from build123d import *

# Parameters (mm, degrees)
SKETCH_1_W          = 106
SKETCH_1_H          = 103
SKETCH_1_W_2        = 102
SKETCH_1_H_2        = 99
EXTRUDE_1_DEPTH     = 25
SKETCH_2_W          = 106
SKETCH_2_H          = 103
EXTRUDE_2_DEPTH     = 1.4
SKETCH_3_R          = 3
SKETCH_3_R_2        = 1.35
EXTRUDE_3_DEPTH     = 5
SKETCH_4_W          = 12.8
SKETCH_4_H          = 11.5
CUT_EXTRUDE_1_DEPTH = 101
FILLET_1_R          = 2
CHAMFER_1_SIZE      = 1
SKETCH_5_R          = 4
SKETCH_5_R_2        = 5
CUT_EXTRUDE_2_DEPTH = 2
SKETCH_6_W          = 3
SKETCH_6_H          = 10
CUT_EXTRUDE_3_DEPTH = 2
SKETCH_8_R          = 1.5
CUT_EXTRUDE_4_DEPTH = 121.470950855
SKETCH_9_R          = 1.5
CUT_EXTRUDE_5_DEPTH = 2
SKETCH_10_W         = 10.5
SKETCH_10_H         = 3
CUT_EXTRUDE_6_DEPTH = 2


with BuildPart() as part:
    # Эскиз1 → Бобышка-Вытянуть1 (new body)
    with BuildSketch(Plane.XY):
        Rectangle(SKETCH_1_W, SKETCH_1_H)
        Rectangle(SKETCH_1_W_2, SKETCH_1_H_2, mode=Mode.SUBTRACT)
    extrude(amount=EXTRUDE_1_DEPTH)

    # Эскиз2 → Бобышка-Вытянуть2 (add)
    with BuildSketch(Plane(origin=(0, 0, 0), x_dir=(-1, 0, 0), z_dir=(0, 0, -1))):
        Rectangle(SKETCH_2_W, SKETCH_2_H)
    extrude(amount=EXTRUDE_2_DEPTH)

    # Эскиз3 → Бобышка-Вытянуть3 (add)
    # profile 1 of 4: a face of its own
    with BuildSketch(Plane.XY):
        with Locations(Location((-45, 39.5, 0), (0, 0, 180))):
            Circle(SKETCH_3_R)
        with Locations((-45, 39.5)):
            Circle(SKETCH_3_R_2, mode=Mode.SUBTRACT)
    # profile 2 of 4: a face of its own
    with BuildSketch(Plane.XY):
        with Locations(Location((45, 39.5, 0), (0, 0, 180))):
            Circle(SKETCH_3_R)
        with Locations((45, 39.5)):
            Circle(SKETCH_3_R_2, mode=Mode.SUBTRACT)
    # profile 3 of 4: a face of its own
    with BuildSketch(Plane.XY):
        with Locations(Location((-45, -43.5, 0), (0, 0, 180))):
            Circle(SKETCH_3_R)
        with Locations((-45, -43.5)):
            Circle(SKETCH_3_R_2, mode=Mode.SUBTRACT)
    # profile 4 of 4: a face of its own
    with BuildSketch(Plane.XY):
        with Locations(Location((45, -43.5, 0), (0, 0, 180))):
            Circle(SKETCH_3_R)
        with Locations((45, -43.5)):
            Circle(SKETCH_3_R_2, mode=Mode.SUBTRACT)
    extrude(amount=EXTRUDE_3_DEPTH)

    # Эскиз4 → Вырез-Вытянуть1 (cut)
    with BuildSketch(Plane.XZ.offset(51.5)):
        with Locations((10.1, 12.35)):
            Rectangle(SKETCH_4_W, SKETCH_4_H)
    extrude(amount=-CUT_EXTRUDE_1_DEPTH, mode=Mode.SUBTRACT)

    # Скругление1
    fillet_1_edges = [part.edges().sort_by_distance(p)[0] for p in [
        (51, -49.5, 12.5),
        (51, 49.5, 12.5),
        (-51, 49.5, 12.5),
        (-51, -49.5, 12.5),
        (53, -51.5, 11.8),
        (-53, -51.5, 11.8),
        (-53, 51.5, 11.8),
        (53, 51.5, 11.8),
    ]]
    fillet(fillet_1_edges, radius=FILLET_1_R)

    # Фаска1
    chamfer_1_edges = [part.edges().sort_by_distance(p)[0] for p in [
        (-51, 0, 0),
        (0, -49.5, 0),
        (51, 0, 0),
        (0, 49.5, 0),
        (50.414213562, -48.914213562, 0),
        (50.414213562, 48.914213562, 0),
        (-50.414213562, 48.914213562, 0),
        (-50.414213562, -48.914213562, 0),
        (-42, 39.5, 0),
        (48, 39.5, 0),
        (-42, -43.5, 0),
        (48, -43.5, 0),
    ]]
    chamfer(chamfer_1_edges, length=CHAMFER_1_SIZE)

    # Эскиз5 → Вырез-Вытянуть2 (cut)
    with BuildSketch(Plane.XZ.offset(51.5)):
        with Locations(Location((32.5, 14.6, 0), (0, 0, 270))):
            Circle(SKETCH_5_R)
        with Locations(Location((-8.3, 14.6, 0), (0, 0, 270))):
            Circle(SKETCH_5_R_2)
    extrude(amount=-CUT_EXTRUDE_2_DEPTH, mode=Mode.SUBTRACT)

    # Эскиз6 → Вырез-Вытянуть3 (cut)
    with BuildSketch(Plane(origin=(53, 0, 0), x_dir=(0, 0, -1), z_dir=(1, 0, 0))):
        with Locations((-23.5, -18.5)):
            Rectangle(SKETCH_6_W, SKETCH_6_H)
        with Locations((-23.5, 7.5)):
            Rectangle(SKETCH_6_W, SKETCH_6_H)
    extrude(amount=-CUT_EXTRUDE_3_DEPTH, mode=Mode.SUBTRACT)

    # Эскиз8 → Вырез-Вытянуть4 (cut, through all)
    with BuildSketch(Plane(origin=(53, 0, 0), x_dir=(0, 0, -1), z_dir=(1, 0, 0))):
        with Locations((-21, 43.5)):
            Circle(SKETCH_8_R)
        with Locations((-21, -43.5)):
            Circle(SKETCH_8_R)
    extrude(amount=-CUT_EXTRUDE_4_DEPTH, mode=Mode.SUBTRACT)

    # Эскиз9 → Вырез-Вытянуть5 (cut)
    with BuildSketch(Plane(origin=(53, 0, 0), x_dir=(0, 0, -1), z_dir=(1, 0, 0))):
        with Locations((-21, -5.5)):
            Circle(SKETCH_9_R)
    extrude(amount=-CUT_EXTRUDE_5_DEPTH, mode=Mode.SUBTRACT)

    # Эскиз10 → Вырез-Вытянуть6 (cut)
    with BuildSketch(Plane(origin=(0, 51.5, 0), x_dir=(1, 0, 0), z_dir=(0, 1, 0))):
        with Locations((9.75, -23.5)):
            Rectangle(SKETCH_10_W, SKETCH_10_H)
    extrude(amount=-CUT_EXTRUDE_6_DEPTH, mode=Mode.SUBTRACT)


solid = part.part
Here's how the part is built. I have some questions about the finished solid (model axes, mm). A direction names the side the tool comes from. Coordinates: 2 decimals unless noted, no trailing zeros. Write each loop counter-clockwise with the first axis right and the second up, starting at its lowest first coordinate (ties: lowest second). Pieces come first, ordered by that corner, then holes. Notation, with made-up numbers: (24, 89.5) - (31, 89.5) arc R26 cw to (31, 120.5) - close; hole circle Ø9 at (43, 49). An arc over 180 degrees is marked (long way). Use one line per item in the form item = value.
1) Suppose I cut it at B-B, the plane y = -5.5. Write out the boundary of the cut face in (x, z), plus the area to 3 significant figures.
Solved:
outline = (-53, -1.4) - (53, -1.4) - (53, 19.5) - (51, 19.5) - (51, 1) - (50, 0) - (-50, 0) - (-51, 1) - (-51, 25) - (-53, 25) - close; (51, 22.5) - (53, 22.5) - (53, 25) - (51, 25) - close
area = 243 mm2
2) Suppose I cut it at A-A, the plane z = 14.6. Write out the boundary of the cut face in (x, y).
Solved:
outline = (-53, -49.5) arc R2 ccw to (-51, -51.5) - (-13.3, -51.5) - (-13.3, -49.5) - (-49, -49.5) arc R2 cw to (-51, -47.5) - (-51, 47.5) arc R2 cw to (-49, 49.5) - (49, 49.5) arc R2 cw to (51, 47.5) - (51, -47.5) arc R2 cw to (49, -49.5) - (36.5, -49.5) - (36.5, -51.5) - (51, -51.5) arc R2 ccw to (53, -49.5) - (53, 49.5) arc R2 ccw to (51, 51.5) - (-51, 51.5) arc R2 ccw to (-53, 49.5) - close; (-3.3, -51.5) - (3.7, -51.5) - (3.7, -49.5) - (-3.3, -49.5) - close; (16.5, -51.5) - (28.5, -51.5) - (28.5, -49.5) - (16.5, -49.5) - close
3) I need wall thicknesses on line 1 (Y direction, x = -45, z = 3.55); line 2 (X direction, y = -22, z = 19.5); line 3 (Y direction, x = -3, z = 13). Which ranges of each line are inside material? Lowest first, please.
Solved:
line_1 = -51.5 to -49.5, -46.5 to -44.85, -42.15 to -40.5, 36.5 to 38.15, 40.85 to 42.5, 49.5 to 51.5
line_2 = -53 to -51, 51 to 53
line_3 = -51.5 to -49.5, 49.5 to 51.5
4) I'm going to push flat-ended pins straight in: P1, Ø4.5, axis at x = -45, y = -43.5, coming from the +Z side; P2, Ø0.6, axis at x = 52, z = 23, coming from the +Y side; P3, Ø1, axis at x = 12.5, y = 11.5, coming from the +Z side. Where does each tip first touch, or does it pass through?
Solved:
P1 = 5
P2 = 51.37
P3 = 0
5) On a 3-axis mill with a long thin cutter (end or side, diameter ignored), from which of +Z, -Z, +X, -X, +Y, -Y can I reach the whole of each face in a straight line? I mean faces 3 (the cylindrical face through (52.01, -5.43, 22.5)), 4 (the flat face through (53, -1, 12)), 5 (the cylindrical face through (36.466, -50.514, 15.121)), 6 (the flat face through (44, -42, 5)), 7 (the flat face through (-53, -1, 12)). Say none if no direction works.
Solved:
face_3 = +X
face_4 = +Z, -Z, +X, +Y, -Y
face_5 = -Y
face_6 = +Z
face_7 = +Z, -Z, -X, +Y, -Y
6) Thinking about a two-plate mould opening in Y: for faces 1 (the cylindrical face through (47.21, -45.53, 2.97)), 2 (the cylindrical face through (-10.215, -50.514, 9.981)), which applies, released by +Y, released by -Y, zero draft, split by the parting line, or undercut?
Solved:
face_1 = undercut
face_2 = zero draft
